Here's how the part is built. I have some questions about the finished solid (model axes, mm). Face numbers are marked on the shaded views. A direction names the side the tool comes from. Give positions to 0.01 mm unless a question says otherwise; leave off trailing zeros. Order: outer loops, then holes, each group sorted by start corner. A loop starts at its lowest first (then second) coordinate and runs counter-clockwise, first axis right, second up. Notation, with made-up numbers: M -22,-39.75 L 11,-39.75 A9 cw 11,-23.75 Z; hole C -39,7 d4. An arc over 180 degrees is marked long. One line per item, written item: value. Start each with the question number.
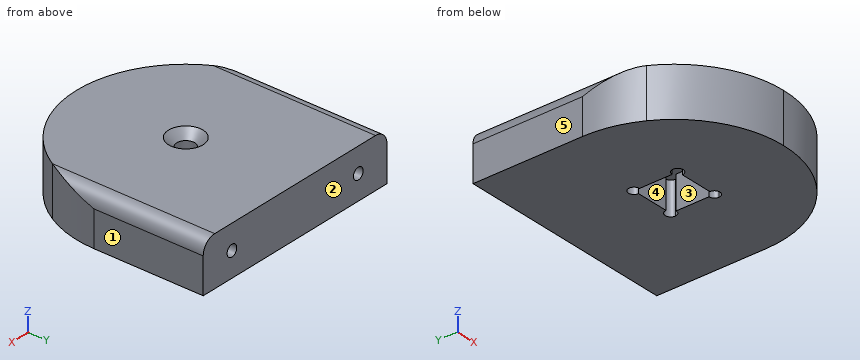
from build123d import *

# Parameters (mm, degrees)
SKETCH1_W                                           = 80
SKETCH1_H                                           = 80
BOSS_EXTRUDE1_DEPTH                                 = 12
SKETCH2_W                                           = 80
SKETCH2_H                                           = 80
SKETCH2_R                                           = 1.5
BOSS_EXTRUDE2_DEPTH                                 = 6
CSK_FOR_M6_COUNTERSUNK_FLAT_HEAD_SCREW1_D           = 6.6
CSK_FOR_M6_COUNTERSUNK_FLAT_HEAD_SCREW1_DEPTH       = 10
CSK_FOR_M6_COUNTERSUNK_FLAT_HEAD_SCREW1_CSINK_D     = 12.6
CSK_FOR_M6_COUNTERSUNK_FLAT_HEAD_SCREW1_CSINK_ANGLE = 90
CSK_FOR_M6_COUNTERSUNK_FLAT_HEAD_SCREW1_TIP         = 1.982840043
FILLET1_R                                           = 5
M5_TAPPED_HOLE1_D                                   = 4.2
M5_TAPPED_HOLE1_DEPTH                               = 12.4
M5_TAPPED_HOLE1_TIP                                 = 1.2618073
CUT_EXTRUDE1_DEPTH                                  = 60.363288319


with BuildPart() as part:
    # Sketch1 → Boss-Extrude1 (new body)
    with BuildSketch(Plane.XY):
        Rectangle(SKETCH1_W, SKETCH1_H)
        with BuildLine():
            Line((6, -8), (-6, -8))
            ThreePointArc((-6, -8), (-9.414213562, -9.414213562), (-8, -6))
            Line((-8, -6), (-8, 6))
            ThreePointArc((-8, 6), (-9.414213562, 9.414213562), (-6, 8))
            Line((-6, 8), (6, 8))
            ThreePointArc((6, 8), (8, 10), (10, 8))
            ThreePointArc((10, 8), (9.414213562, 6.585786438), (8, 6))
            Line((8, 6), (8, -6))
            ThreePointArc((8, -6), (9.414213562, -6.585786438), (10, -8))
            ThreePointArc((10, -8), (8, -10), (6, -8))
        make_face(mode=Mode.SUBTRACT)
    extrude(amount=BOSS_EXTRUDE1_DEPTH)

    # Sketch2 → Boss-Extrude2 (add)
    with BuildSketch(Plane.XY.offset(12)):
        Rectangle(SKETCH2_W, SKETCH2_H)
        Circle(SKETCH2_R, mode=Mode.SUBTRACT)
    extrude(amount=BOSS_EXTRUDE2_DEPTH)

    # CSK for M6 Countersunk Flat Head Screw1
    with Locations(Plane.XY.offset(18)):
        with Locations((0, 0)):
            CounterSinkHole(CSK_FOR_M6_COUNTERSUNK_FLAT_HEAD_SCREW1_D / 2, CSK_FOR_M6_COUNTERSUNK_FLAT_HEAD_SCREW1_CSINK_D / 2, depth=CSK_FOR_M6_COUNTERSUNK_FLAT_HEAD_SCREW1_DEPTH, counter_sink_angle=CSK_FOR_M6_COUNTERSUNK_FLAT_HEAD_SCREW1_CSINK_ANGLE)
            with Locations((0, 0, -(CSK_FOR_M6_COUNTERSUNK_FLAT_HEAD_SCREW1_DEPTH + CSK_FOR_M6_COUNTERSUNK_FLAT_HEAD_SCREW1_TIP / 2))):  # 118° drill point
                Cone(0, CSK_FOR_M6_COUNTERSUNK_FLAT_HEAD_SCREW1_D / 2, CSK_FOR_M6_COUNTERSUNK_FLAT_HEAD_SCREW1_TIP, mode=Mode.SUBTRACT)

    # Fillet1
    fillet1_edges = [part.edges().sort_by_distance(p)[0] for p in [
        (-40, 0, 18),
        (40, 0, 18),
    ]]
    fillet(fillet1_edges, radius=FILLET1_R)

    # M5 Tapped Hole1
    with Locations(Plane(origin=(0, 40, 0), x_dir=(1, 0, 0), z_dir=(0, 1, 0))):
        with Locations((-27.5, -9), (27.5, -9.012634245)):
            Hole(M5_TAPPED_HOLE1_D / 2, depth=M5_TAPPED_HOLE1_DEPTH)
            with Locations((0, 0, -(M5_TAPPED_HOLE1_DEPTH + M5_TAPPED_HOLE1_TIP / 2))):  # 118° drill point
                Cone(0, M5_TAPPED_HOLE1_D / 2, M5_TAPPED_HOLE1_TIP, mode=Mode.SUBTRACT)

    # Sketch7 → Cut-Extrude1 (cut, through all)
    with BuildSketch(Plane.XY.offset(18)):
        with BuildLine():
            ThreePointArc((0, -40), (-20.315060063, -34.457195687), (-35, -19.364916731))
            Line((-35, -19.364916731), (-35, -40))
            Line((-35, -40), (0, -40))
        make_face()
        with BuildLine():
            ThreePointArc((-35, -19.364916731), (-38.729833462, -10), (-40, 0))
            Line((-40, 0), (-40, -40))
            Line((-40, -40), (-35, -40))
            Line((-35, -40), (-35, -19.364916731))
        make_face()
        with BuildLine():
            ThreePointArc((35, -19.364916731), (20.315060063, -34.457195687), (0, -40))
            Line((0, -40), (35, -40))
            Line((35, -40), (35, -19.364916731))
        make_face()
        with BuildLine():
            Line((35, -19.364916731), (35, -40))
            Line((35, -40), (40, -40))
            Line((40, -40), (40, 0))
            ThreePointArc((40, 0), (38.729833462, -10), (35, -19.364916731))
        make_face()
    extrude(amount=-CUT_EXTRUDE1_DEPTH, mode=Mode.SUBTRACT)


solid = part.part
Item 1: We'd pull the mould along Y, two halves only. Please class the marked faces 1, 2 and 3: +Y half, -Y half, draft (parallel to the pull), parting line (faces both ways), or undercut.
Item 2: I want a section at B-B on x = -15. Write out the boundary of the cut face in (y, z).
Item 3: For the marked faces 4 and 5, which set-ups out of +Z, -Z, +X, -X, +Y, -Y let a thin tool reach every point of the face, with its end or its side?
Item 4: I want a section at A-A on y = -15.5. Write out the boundary of the cut face in (x, z).
Item 5: I want a section at C-C on x = 20.5. Write out the boundary of the cut face in (y, z).
Item 6: Will these pins go through, and if not, where does the flat tip stop? P1, Ø2.5, axis at x = 27.5, z = 9.01, coming from the -Y side; P2, Ø6.5, axis at x = -8, y = -8, coming from the -Z side; P3, Ø1.5, axis at y = -13.5, z = 6, coming from the -X side; P4, Ø6, axis at x = -2.5, y = 4, coming from the -Z side.
Item 7: Please list where these lines run through material, in increasing order: probe 1 along X at (y, z) = (36.5, 9); probe 2 along X at (y, z) = (3, 11.25); probe 3 along Z at (x, y) = (-27, 33). Write a range as [from, to].
Answer below:
1. face 1: draft
1. face 2: +Y half
1. face 3: undercut
2. outline: M -37.08,0 L 40,0 L 40,18 L -37.08,18 Z
3. face 4: -Z
3. face 5: +Z, -Z, -X, +Y, -Y
4. outline: M -36.87,0 L 36.87,0 L 36.87,17.64 A5 ccw 35,18 L -35,18 A5 ccw -36.87,17.64 Z
5. outline: M -34.35,0 L 40,0 L 40,18 L -34.35,18 Z
6. P1: stops at y = -30.18
6. P2: stops at z = 0
6. P3: stops at x = -37.91
6. P4: stops at z = 12
7. probe 1: x = [-40, -29.6], [-25.4, 25.4], [29.6, 40]
7. probe 2: x = [-40, -8], [8, 40]
7. probe 3: z = [0, 6.96], [11.04, 18]
